The listing builds one solid part. Answer for the finished solid, in the listing's coordinates (mm). A direction names the side the tool comes from. Give positions to 0.01 mm unless a question says otherwise; leave off trailing zeros. Order: outer loops, then holes, each group sorted by start corner. A loop starts at its lowest first (then second) coordinate and runs counter-clockwise, first axis right, second up. Notation, with made-up numbers: M 78,77.25 L 93,77.25 A25 ccw 93,113.25 Z; hole C -23,78 d11. An arc over 180 degrees is marked long. Answer as a JSON object with one key per item and string values. Group by question number.
```python
from build123d import *

# Parameters (mm, degrees)
SKETCH1_R             = 3
SKETCH1_R_2           = 7.5
BOSS_EXTRUDE1_DEPTH   = 3
CORTAR_EXTRUIR1_DEPTH = 85.905830189
CROQUIS2_R            = 1.5
CORTAR_EXTRUIR2_DEPTH = 85.905830189


with BuildPart() as part:
    # Sketch1 → Boss-Extrude1 (new body)
    with BuildSketch(Plane(origin=(0, 0, 0), x_dir=(1, 0, 0), z_dir=(0, 1, 0))):
        with BuildLine():
            Line((-10.606601718, 60), (-10.606601718, -10.606601718))
            Line((-10.606601718, -10.606601718), (60, -10.606601718))
            Line((60, -10.606601718), (60, 0))
            ThreePointArc((60, 0), (42.426406871, 42.426406871), (0, 60))
            Line((0, 60), (-10.606601718, 60))
        make_face()
        with Locations(Location((0, 0, 0), (0, 0, 270))):
            Circle(SKETCH1_R, mode=Mode.SUBTRACT)
        with Locations(Location((50, 0, 0), (0, 0, 270))):
            Circle(SKETCH1_R_2, mode=Mode.SUBTRACT)
    extrude(amount=BOSS_EXTRUDE1_DEPTH)

    # Croquis1 → Cortar-Extruir1 (cut, through all)
    with BuildSketch(Plane(origin=(0, 3, 0), x_dir=(1, 0, 0), z_dir=(0, 1, 0))):
        with BuildLine():
            ThreePointArc((0, 10.606601718), (0.38870443, 10.59947682), (0.776886642, 10.5781117))
            Line((0.776886642, 10.5781117), (38.575945262, 10.5781117))
            ThreePointArc((38.575945262, 10.5781117), (24.257736209, 31.805066169), (0, 40))
            Line((0, 40), (0, 10.606601718))
        make_face()
        with BuildLine():
            ThreePointArc((0, -10.606601718), (-7.5, -7.5), (-10.606601718, 0))
            Line((-10.606601718, 0), (-10.606601718, -10.606601718))
            Line((-10.606601718, -10.606601718), (0, -10.606601718))
        make_face()
    extrude(amount=-CORTAR_EXTRUIR1_DEPTH, mode=Mode.SUBTRACT)

    # Croquis2 → Cortar-Extruir2 (cut, through all)
    with BuildSketch(Plane(origin=(0, 3, 0), x_dir=(1, 0, 0), z_dir=(0, 1, 0))):
        with Locations(Location((8, 0, 0), (0, 0, 270))):
            Circle(CROQUIS2_R)
        with Locations(Location((0, -8, 0), (0, 0, 270))):
            Circle(CROQUIS2_R)
        with Locations(Location((-8, 0, 0), (0, 0, 270))):
            Circle(CROQUIS2_R)
        with Locations(Location((0, 8, 0), (0, 0, 270))):
            Circle(CROQUIS2_R)
    extrude(amount=-CORTAR_EXTRUIR2_DEPTH, mode=Mode.SUBTRACT)


solid = part.part
```
Item 1: A tool of negligible diameter and unlimited length cuts with its end or side. For faces 5 (the flat face through (-10.607, 1, -30)), 6 (the flat face through (19, 2, -10.578)), from which of +Z, -Z, +X, -X, +Y, -Y can it reach the whole face along a straight path? Write none if from no direction.
Item 2: Consider probe 1 along X at (y, z) = (0.55, 2); probe 2 along X at (y, z) = (1.95, 8); probe 3 along Z at (x, y) = (47, 2.45). Determine where each line is inside the solid, lowest interval first. Write a range as from..to.
Item 3: Section C-C (z = -37) is taken. Determine the outline of the cut face in (x, y), and give its area (3 significant figures).
Item 4: Determine the mould class of faces 1 (the cylindrical face through (0.9, 1.48, 2.86)), 2 (the cylindrical face through (24.55, 1.52, -31.58)), 3 (the cylindrical face through (42.89, 1.48, -41.96)), 4 (the flat face through (24, 3, -33)) for opening direction X: released by +X, released by -X, zero draft, split by the parting line, or undercut.
Item 5: Section B-B (x = 24.5) is taken. Determine the outline of the cut face in (y, z).
Item 6: Section D-D (x = 8) is taken. Determine the outline of the cut face in (y, z).
Item 7: Section A-A (y = 2) is taken. Determine the outline of the cut face in (x, z).
Values found:
{
 "1": {"face 5": "+Z, -Z, -X, +Y, -Y", "face 6": "+Y, -Y"},
 "2": {"probe 1": "x = -10.42..-2.24, 2.24..42.77, 57.23..60", "probe 2": "x = -6.96..-1.5, 1.5..60", "probe 3": "z = -37.3..-6.87, 6.87..10.61"},
 "3": {"outline": "M -10.61,0 L 0,0 L 0,3 L -10.61,3 Z; M 15.2,0 L 47.23,0 L 47.23,3 L 15.2,3 Z", "area": "128 mm^2"},
 "4": {"face 1": "undercut", "face 2": "undercut", "face 3": "released by +X", "face 4": "zero draft"},
 "5": {"outline": "M 0,-54.77 L 3,-54.77 L 3,-31.62 L 0,-31.62 Z; M 0,-10.58 L 3,-10.58 L 3,10.61 L 0,10.61 Z"},
 "6": {"outline": "M 0,-59.46 L 3,-59.46 L 3,-39.19 L 0,-39.19 Z; M 0,-10.58 L 3,-10.58 L 3,-1.5 L 0,-1.5 Z; M 0,1.5 L 3,1.5 L 3,10.61 L 0,10.61 Z"},
 "7": {"outline": "M -10.61,-60 L 0,-60 A60 ccw 60,0 L 60,10.61 L 0,10.61 A10.61 ccw -10.61,0 Z; hole C -8,0 d3; hole C 0,0 d6; hole C 0,-8 d3; hole C 0,8 d3; hole M 0,-40 A40 ccw 38.58,-10.58 L 0.78,-10.58 A10.61 cw 0,-10.61 Z; hole C 8,0 d3; hole C 50,0 d15"}
}
